The model under review builds one solid part; all positions refer to its coordinate system, in mm. A direction names the side the tool comes from. Coordinates: 2 decimals unless noted, no trailing zeros. Order: outer loops, then holes, each group sorted by start corner. A loop starts at its lowest first (then second) coordinate and runs counter-clockwise, first axis right, second up. Notation, with made-up numbers: (10, 40.5) -> (28, 40.5) arc R17 ccw to (28, 53.5) -> close; hole circle Ø2 at (-16.5, 88.25). An arc over 180 degrees is marked (long way). Use one line per item in the form item = value.
from build123d import *

# Parameters (mm, degrees)
BOSS_EXTRUDE1_DEPTH = 200
CUT_EXTRUDE1_DEPTH  = 180
SKETCH6_W           = 360
SKETCH6_H           = 160
CUT_EXTRUDE2_DEPTH  = 671.794129466
SKETCH7_W           = 101.456658586
SKETCH7_H           = 160
CUT_EXTRUDE3_DEPTH  = 30
SKETCH8_W           = 101.456658586
SKETCH8_H           = 160
CUT_EXTRUDE4_DEPTH  = 30
SKETCH9_W           = 101.37152343
SKETCH9_H           = 160
CUT_EXTRUDE5_DEPTH  = 30
SKETCH10_W          = 101.371523429
SKETCH10_H          = 160
CUT_EXTRUDE6_DEPTH  = 30
SKETCH11_W          = 159.950111148
SKETCH11_H          = 160
CUT_EXTRUDE7_DEPTH  = 749.274973447


with BuildPart() as part:
    # Sketch1 → Boss-Extrude1 (new body)
    with BuildSketch(Plane(origin=(0, 0, 0), x_dir=(0, 1, 0), z_dir=(0, 0, 1))):
        Polygon((-400, 0), (-499.964762884, 99.964762884), (-499.964762884, 299.914874032), (-400, 400), (0, 400), (99.964762884, 299.914874032), (99.964762884, 99.964762884), (0, 0), align=None)
    extrude(amount=BOSS_EXTRUDE1_DEPTH)

    # Sketch4 → Cut-Extrude1 (cut)
    with BuildSketch(Plane.XY.offset(200)):
        Polygon((-30, -387.573593129), (-30, -12.426406871), (-112.391169755, 69.964762884), (-287.499039265, 69.964762884), (-370, -12.43698161), (-370, -387.56301839), (-287.499039265, -469.964762884), (-112.391169755, -469.964762884), align=None)
    extrude(amount=-CUT_EXTRUDE1_DEPTH, mode=Mode.SUBTRACT)

    # Sketch6 → Cut-Extrude2 (cut, through all)
    with BuildSketch(Plane(origin=(-400, 0, 0), x_dir=(0, -1, 0), z_dir=(-1, 0, 0))):
        with Locations((200, 100)):
            Rectangle(SKETCH6_W, SKETCH6_H)
    extrude(amount=-CUT_EXTRUDE2_DEPTH, mode=Mode.SUBTRACT)

    # Sketch7 → Cut-Extrude3 (cut)
    with BuildSketch(Plane(origin=(-199.759333952, 199.9998552, 0), x_dir=(-0.7075320947633997, -0.7066812116362764, 0), z_dir=(-0.7066812116362764, 0.7075320947633997, 0))):
        with Locations((212.284508612, 100)):
            Rectangle(SKETCH7_W, SKETCH7_H)
    extrude(amount=-CUT_EXTRUDE3_DEPTH, mode=Mode.SUBTRACT)

    # Sketch8 → Cut-Extrude4 (cut)
    with BuildSketch(Plane(origin=(-399.759189151, -400.240521248, 0), x_dir=(0.7075320947633943, -0.7066812116362818, 0), z_dir=(-0.7066812116362818, -0.7075320947633943, 0))):
        with Locations((70.387976042, 100)):
            Rectangle(SKETCH8_W, SKETCH8_H)
    extrude(amount=-CUT_EXTRUDE4_DEPTH, mode=Mode.SUBTRACT)

    # Sketch9 → Cut-Extrude5 (cut)
    with BuildSketch(Plane(origin=(0, 0, 0), x_dir=(-0.7071067811865487, 0.7071067811865465, 0), z_dir=(0.7071067811865465, 0.7071067811865487, 0))):
        with Locations((70.685761715, 100)):
            Rectangle(SKETCH9_W, SKETCH9_H)
    extrude(amount=-CUT_EXTRUDE5_DEPTH, mode=Mode.SUBTRACT)

    # Sketch10 → Cut-Extrude6 (cut)
    with BuildSketch(Plane(origin=(200, -200, 0), x_dir=(0.7071067811865439, 0.7071067811865511, 0), z_dir=(0.7071067811865511, -0.7071067811865439, 0))):
        with Locations((-353.52847419, 100)):
            Rectangle(SKETCH10_W, SKETCH10_H)
    extrude(amount=-CUT_EXTRUDE6_DEPTH, mode=Mode.SUBTRACT)

    # Sketch11 → Cut-Extrude7 (cut, through all)
    with BuildSketch(Plane.XZ.offset(499.964762884)):
        with Locations((-199.939818458, 100)):
            Rectangle(SKETCH11_W, SKETCH11_H)
    extrude(amount=-CUT_EXTRUDE7_DEPTH, mode=Mode.SUBTRACT)


solid = part.part
Item 1: We need section C-C (z = 84.5). State how many separate pieces and enclosed holes the cut face has, plus the area to 3 significant figures.
Results found:
separate_pieces = 8
enclosed_holes = 0
area = 6,620 mm²
Item 2: To check wall thickness, follow L1, parallel to Z at x = -375, y = -188; L2, parallel to Z at x = -357, y = -12.5; L3, parallel to Y at x = -294, z = 41. State the ranges of each line that lie inside material, in increasing order. Write a range as from..to.
Results found:
L1 = 0..20, 180..200
L2 = 0..20
L3 = -499.96..-465.74, 65.74..99.96
Item 3: Draft analysis for pull direction X (two halves, no side actions). For faces 6 (the face through (-200, 69.965, 184)), 7 (the face through (-15, -20, 99)), 8 (the face through (-279.915, 85, 99)), 9 (the face through (-96.281, 75.365, 98.88)), state which applies: released by +X, released by -X, zero draft, split by the parting line, or undercut.
Results found:
face_6 = undercut
face_7 = zero draft
face_8 = undercut
face_9 = released by +X
Item 4: We need section A-A (x = -135). Write out the cut boundary in (y, z), plus the area to 3 significant figures.
Results found:
outline = (-499.96, 0) -> (99.96, 0) -> (99.96, 20) -> (-499.96, 20) -> close; (-499.96, 180) -> (-469.96, 180) -> (-469.96, 200) -> (-499.96, 200) -> close; (69.96, 180) -> (99.96, 180) -> (99.96, 200) -> (69.96, 200) -> close
area = 13,200 mm²
Item 5: Clearance check with flat-ended pins moving along their axes: pin 1 (6 mm diameter, centred on x = -121.5, y = -329, fed in from -Z); pin 2 (9 mm diameter, centred on y = -488.5, z = 122.5, fed in from -X); pin 3 (1.5 mm diameter, centred on x = -114, y = -45.5, fed in from +Z); pin 4 (24 mm diameter, centred on y = 89, z = 89, fed in from +X). State where each tip first meets the part, or that it passes through.
Results found:
pin_1 = 0
pin_2 = -314.07
pin_3 = 20
pin_4 = -85.82
Item 6: Tool access review of faces 1 (the face through (-385, -197, 180)), 2 (the face through (-201, 85, 180)), 3 (the face through (-24.6, 3.684, 98.88)), 4 (the face through (-339, 40, 180)), 5 (the face through (-200, -469.965, 184)): name each direction out of +Z, -Z, +X, -X, +Y, -Y from which nothing blocks a thin tool from reaching the whole face with its end or side.
Results found:
face_1 = +X, -X
face_2 = +Y, -Y
face_3 = +Y
face_4 = none
face_5 = +Z
Item 7: We need section B-B (y = -74.5). Write out the cut boundary in (x, z), plus the area to 3 significant figures.
Results found:
outline = (-400, 0) -> (0, 0) -> (0, 20) -> (-400, 20) -> close; (-400, 180) -> (-370, 180) -> (-370, 200) -> (-400, 200) -> close; (-30, 180) -> (0, 180) -> (0, 200) -> (-30, 200) -> close
area = 9,200 mm²
